Autodesk Inventor part; units mm, degrees
ref_plane "YZ Plane" through (0, 0, 0) normal (1, 0, 0) x (0, 1, 0)
ref_plane "XZ Plane" through (0, 0, 0) normal (0, 1, 0) x (-1, 0, 0)
ref_plane "XY Plane" through (0, 0, 0) normal (0, 0, 1) x (1, 0, 0)
sketch "Sketch1" plane through (0, 0, 0) normal (0, 1, 0) x (-1, 0, 0)
  circle A0 centre (0, 0) radius 1.5
  line L0 (-0.7211, -2.912) -> (-2.8825, -0.8315)
  line L1 (-2.8825, -0.8315) -> (-2.1614, 2.0805)
  line L2 (-2.1614, 2.0805) -> (0.7211, 2.912)
  line L3 (0.7211, 2.912) -> (2.8825, 0.8315)
  line L4 (2.8825, 0.8315) -> (2.1614, -2.0805)
  line L5 (2.1614, -2.0805) -> (-0.7211, -2.912)
  dimension "d0" = 3
  dimension "d1" = 6
extrude "Extrusion1" add sketch "Sketch1" along normal blind 40
thread "Thread1"
thread "Thread2"
properties part number "Spacer40"
Geometry check sheet. Reference: the model listing, model coordinates, mm. Coordinates: 2 decimals unless noted, no trailing zeros. Order: outer loops, then holes, each group sorted by start corner. A loop starts at its lowest first (then second) coordinate and runs counter-clockwise, first axis right, second up.
Item 1: Scan lines: line 1 along Z through (x, y) = (0, 23.5); line 2 along X through (y, z) = (5, -1.25); line 3 along Z through (x, y) = (-0.2, 33.5). Record each from-to range of solid material in increasing order.
Item 2: Section check A-A (y = 23). Enter the section's corners in (x, z), plus the area to 3 significant figures.
Item 3: Section check B-B (x = 0). Enter the section's corners in (y, z).
Item 4: Mould release check, pull along X, two halves, no side actions. Record for faces 1 (the cylindrical face through (1.5, 19.72, -0.07)), 2 (the flat face through (-1.787, 19.72, 1.886)), 3 (the flat face through (2.53, 19.72, 0.6)): released by +X, released by -X, zero draft, split by the parting line, or undercut.
Item 5: Depth check by flat-ended pin: pin 1 (1.5 mm diameter, centred on y = 16.5, z = 0.5, fed in from -X); pin 2 (1 mm diameter, centred on y = 27.5, z = -1.5, fed in from -X); pin 3 (3 mm diameter, centred on y = 13.5, z = -1, fed in from -X). Enter the tip coordinate at first touch or a pass-through.
Item 6: Section check C-C (z = -0.35). Enter the section's corners in (x, y).
Check sheet entries:
1. line 1: z = -2.7 to -1.5, 1.5 to 2.7
1. line 2: x = -2.37 to -0.83, 0.83 to 2.45
1. line 3: z = -2.65 to -1.49, 1.49 to 2.76
2. outline: (-2.88, 0.83) - (-2.16, -2.08) - (0.72, -2.91) - (2.88, -0.83) - (2.16, 2.08) - (-0.72, 2.91) - close; hole circle Ø3 at (0, 0)
2. area: 16.3 mm2
3. outline: (0, -2.7) - (40, -2.7) - (40, -1.5) - (0, -1.5) - close; (0, 1.5) - (40, 1.5) - (40, 2.7) - (0, 2.7) - close
4. face 1: undercut
4. face 2: released by -X
4. face 3: released by +X
5. pin 1: stops at x = -2.88
5. pin 2: stops at x = -2.43
5. pin 3: stops at x = -2.8
6. outline: (-2.59, 0) - (-1.46, 0) - (-1.46, 40) - (-2.59, 40) - close; (1.46, 0) - (2.76, 0) - (2.76, 40) - (1.46, 40) - close
